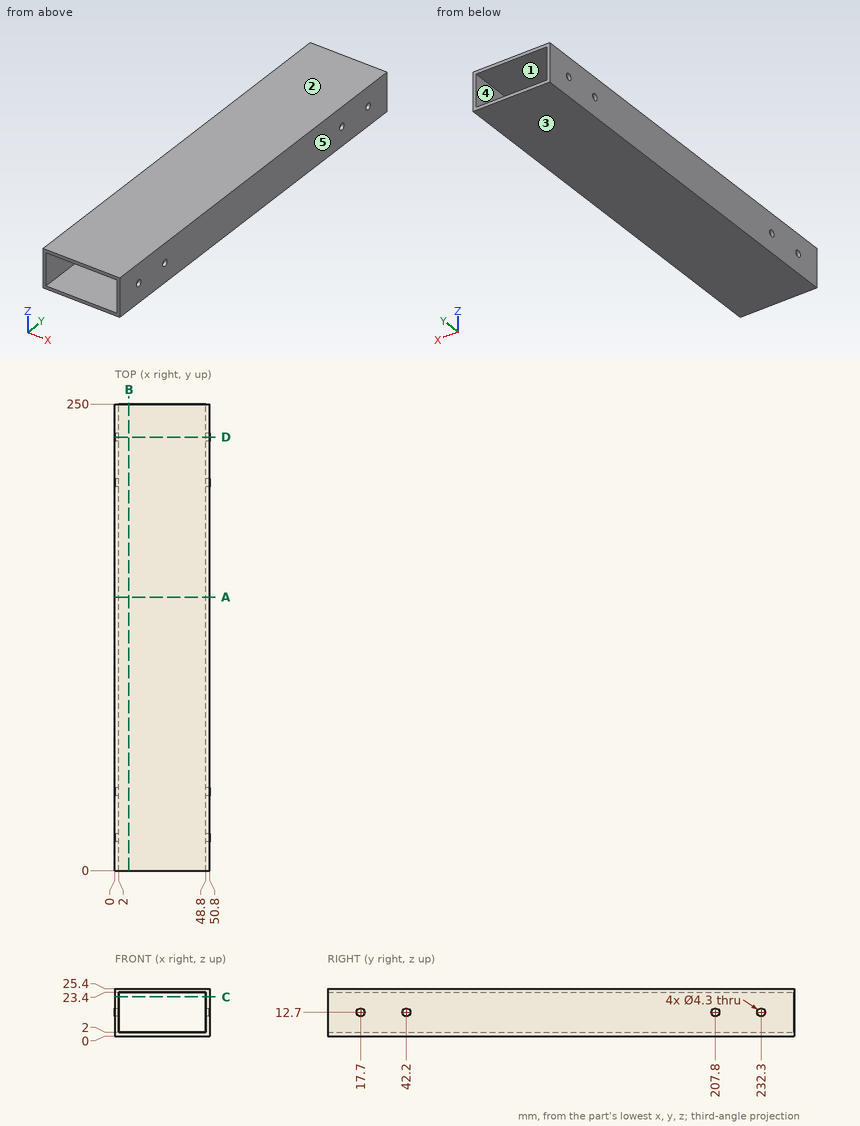
The drawing under review shows one solid part. Ordinate dimensions are in mm from its lowest x, y, z. A direction names the side the tool comes from. Coordinates: 2 decimals unless noted, no trailing zeros. Order: outer loops, then holes, each group sorted by start corner. A loop starts at its lowest first (then second) coordinate and runs counter-clockwise, first axis right, second up. Notation, with made-up numbers: (86.25, 7) -> (140.25, 7) arc R29 cw to (140.25, 35) -> close; hole circle Ø10 at (46.5, -16). An arc over 180 degrees is marked (long way). Answer in a Markdown table with one row per item. Add a question column.
Item 1: We need section B-B on x = 7.5. Write out the cut boundary in (y, z).
Item 2: Machinability: for the marked faces 1 and 2, which of the approach directions +Z, -Z, +X, -X, +Y, -Y give a long, thin tool a straight path to every point of the face, cutting with its end or side? Answer none if there is none.
Item 3: We need section C-C on z = 21. Write out the cut boundary in (x, y), plus the area to 3 significant figures.
Item 4: Clearance check with a flat-ended pin moving along its axis: pin 1 (4 mm diameter, centred on y = 42.2, z = 12.7, fed in from +X). State where the tip first meets the part, or that it passes through.
Item 5: Mouldability with a two-part tool opening along Z and no side actions: class the marked faces 3, 4 and 5 as +Z half, -Z half, draft (parallel to the pull), parting line (faces both ways), or undercut.
Item 6: To check wall thickness, follow probe 1 along Y at (x, z) = (49.75, 12.7); probe 2 along X at (y, z) = (112, 2.5); probe 3 along Z at (x, y) = (37.5, 74). State the ranges of each line that lie inside material, in increasing order.
Item 7: We need section D-D on y = 232.3. Write out the cut boundary in (x, z).
Item 8: We need section A-A on y = 146.5. Write out the cut boundary in (x, z).
Final values:
| question | item | result |
|---|---|---|
| 1 | outline | (0, 0) -> (250, 0) -> (250, 2) -> (0, 2) -> close; (0, 23.4) -> (250, 23.4) -> (250, 25.4) -> (0, 25.4) -> close |
| 2 | face 1 | +Y, -Y |
| 2 | face 2 | +Z, +X, -X, +Y, -Y |
| 3 | outline | (0, 0) -> (2, 0) -> (2, 250) -> (0, 250) -> close; (48.8, 0) -> (50.8, 0) -> (50.8, 250) -> (48.8, 250) -> close |
| 3 | area | 1,000 mm2 |
| 4 | pin 1 | passes through |
| 5 | face 3 | -Z half |
| 5 | face 4 | undercut |
| 5 | face 5 | draft |
| 6 | probe 1 | y = 0 to 15.55, 19.85 to 40.05, 44.35 to 205.65, 209.95 to 230.15, 234.45 to 250 |
| 6 | probe 2 | x = 0 to 2, 48.8 to 50.8 |
| 6 | probe 3 | z = 0 to 2, 23.4 to 25.4 |
| 7 | outline | (0, 0) -> (50.8, 0) -> (50.8, 10.55) -> (48.8, 10.55) -> (48.8, 2) -> (2, 2) -> (2, 10.55) -> (0, 10.55) -> close; (0, 14.85) -> (2, 14.85) -> (2, 23.4) -> (48.8, 23.4) -> (48.8, 14.85) -> (50.8, 14.85) -> (50.8, 25.4) -> (0, 25.4) -> close |
| 8 | outline | (0, 0) -> (50.8, 0) -> (50.8, 25.4) -> (0, 25.4) -> close; hole (2, 2) -> (48.8, 2) -> (48.8, 23.4) -> (2, 23.4) -> close |
